The model under review builds one solid part; all positions refer to its coordinate system, in mm. A direction names the side the tool comes from. Give positions to 0.01 mm unless a question says otherwise; leave off trailing zeros. Order: outer loops, then holes, each group sorted by start corner. A loop starts at its lowest first (then second) coordinate and runs counter-clockwise, first axis right, second up. Notation, with made-up numbers: M -15.5,29 L 5.5,29 A29 cw 5.5,66 Z; hole C 83.25,-9.5 d2. An arc over 180 degrees is marked long. One line per question, with ' | ' between items. Start each with the question number.
1. We need section A-A on z = -17. Write out the cut boundary in (x, y).
2. Wall thickness on L1, parallel to Z at x = 85, y = 4.25; L2, parallel to Z at x = 47.5, y = 38; L3, parallel to X at y = 105.5, z = -13 (3 decimals): over which ranges is each line inside the solid? List them lowest first.
3. The part is to be moulded in two halves that separate along Z. For faces 1 (the face through (48, 42, 0)), 2 (the face through (86.63, 7.6, 27.68)), 3 (the face through (40, 34, -5)), say which applies: +Z half, -Z half, draft (parallel to the pull), parting line (faces both ways), or undercut.
4. We need section B-B on y = 105. Write out the cut boundary in (x, z).
5. For faces 4 (the face through (-25.646, 49.91, 11.811)), 5 (the face through (7, 41, -50)), 6 (the face through (67, 15, 12)), 7 (the face through (-95.49, 7.6, 45.72)), 8 (the face through (25.38, 50.9, 11.81)), list the 3-axis set-ups (+Z, -Z, +X, -X, +Y, -Y) from which the entire face can be reached by the end or side of a thin tool; tool diameter is ignored.
6. We need section C-C on x = 0. Write out the cut boundary in (y, z), then the cut area to 3 significant figures.
7. We need section D-D on x = -50. Write out the cut boundary in (y, z), then the cut area to 3 significant figures.
8. Insertion check: P1, Ø10, axis at x = 53.5, z = -1, coming from the +Y side; P2, Ø19.5, axis at x = 52, z = -5, coming from the +Y side; P3, Ø2, axis at y = 110.5, z = 30, coming from the -X side; P4, Ø17, axis at x = -85, z = -35, coming from the -Y side. Each pin has a flat end and moves straight along its axis. Give the tip position at first contact, or say it passes through.
```python
from build123d import *

# Parameters (mm, degrees)
SKETCH1_R           = 12.5
BOSS_EXTRUDE1_DEPTH = 50
FILLET1_R           = 15
SKETCH2_R           = 7.5
CUT_EXTRUDE1_DEPTH  = 161.390149323
RIB1_REACH          = 173.464
SKETCH3_WALL_W      = 422.202630092
SKETCH3_WALL_H      = 10


with BuildPart() as part:
    # Sketch1 → Boss-Extrude1 (new, symmetric)
    with BuildSketch(Plane.XY):
        with BuildLine():
            Line((-35, 15), (-16.025916537, 85.81224351))
            ThreePointArc((-16.025916537, 85.81224351), (0, 130), (16.025916537, 85.81224351))
            Line((16.025916537, 85.81224351), (35, 15))
            Line((35, 15), (100, 15))
            Line((100, 15), (100, 0))
            Line((100, 0), (-100, 0))
            Line((-100, 0), (-100, 15))
            Line((-100, 15), (-35, 15))
        make_face()
        with Locations((0, 105)):
            Circle(SKETCH1_R, mode=Mode.SUBTRACT)
    extrude(amount=BOSS_EXTRUDE1_DEPTH, both=True)

    # Fillet1
    fillet1_edges = [part.edges().sort_by_distance(p)[0] for p in [
        (100, 7.5, -50),
        (-100, 7.5, -50),
        (100, 7.5, 50),
        (-100, 7.5, 50),
    ]]
    fillet(fillet1_edges, radius=FILLET1_R)

    # Sketch2 → Cut-Extrude1 (cut, through all)
    with BuildSketch(Plane(origin=(0, 15, 0), x_dir=(1, 0, 0), z_dir=(0, 1, 0))):
        with Locations(Location((-85, 35, 0), (0, 0, 180))):
            Circle(SKETCH2_R)
        with Locations(Location((-85, -35, 0), (0, 0, 180))):
            Circle(SKETCH2_R)
        with Locations(Location((85, 35, 0), (0, 0, 180))):
            Circle(SKETCH2_R)
        with Locations(Location((85, -35, 0), (0, 0, 180))):
            Circle(SKETCH2_R)
    extrude(amount=-CUT_EXTRUDE1_DEPTH, mode=Mode.SUBTRACT)

    # Sketch3 wall → Rib1 (add, up to next)
    with BuildSketch(Plane(origin=(47.679491924, 42.320508076, 0), x_dir=(-0.707106781187, 0.707106781187, 0), z_dir=(-0.707106781187, -0.707106781187, 0)), mode=Mode.PRIVATE) as rib1_sk1:
        Rectangle(SKETCH3_WALL_W, SKETCH3_WALL_H)
    rib1_tool1 = extrude(rib1_sk1.sketch, amount=RIB1_REACH, mode=Mode.PRIVATE) - part.part
    rib1 = rib1_tool1.solids().sort_by_distance((47.679491924, 42.320508076, 0))[0]
    add(rib1)

    # Mirror1: Rib1 across plane
    add(rib1.mirror(Plane(origin=(0, 0, 0), x_dir=(0, 0, 1), z_dir=(1, 0, 0))))


solid = part.part
```
Entries:
1) outline: M -100,0 L 100,0 L 100,15 L 35,15 L 16.03,85.81 A25 ccw long -16.03,85.81 L -35,15 L -100,15 Z; hole C 0,105 d25
2) L1: z = -50 to -42.5, -27.5 to 27.5, 42.5 to 50 | L2: z = -5 to 5 | L3: x = -24.995 to -12.49, 12.49 to 24.995
3) face 1: draft | face 2: undercut | face 3: -Z half
4) outline: M -25,-50 L -12.5,-50 L -12.5,50 L -25,50 Z; M 12.5,-50 L 25,-50 L 25,50 L 12.5,50 Z
5) face 4: -X | face 5: -Z, +X, -X, +Y, -Y | face 6: +X, +Y | face 7: +Z, -X, +Y, -Y | face 8: +X
6) outline: M 0,-50 L 92.5,-50 L 92.5,50 L 0,50 Z; M 117.5,-50 L 130,-50 L 130,50 L 117.5,50 Z | area: 10,500 mm^2
7) outline: M 0,-50 L 15,-50 L 15,-5 L 40,-5 L 40,5 L 15,5 L 15,50 L 0,50 Z | area: 1,750 mm^2
8) P1: stops at y = 41.5 | P2: stops at y = 47.75 | P3: stops at x = -24.59 | P4: stops at y = 0
